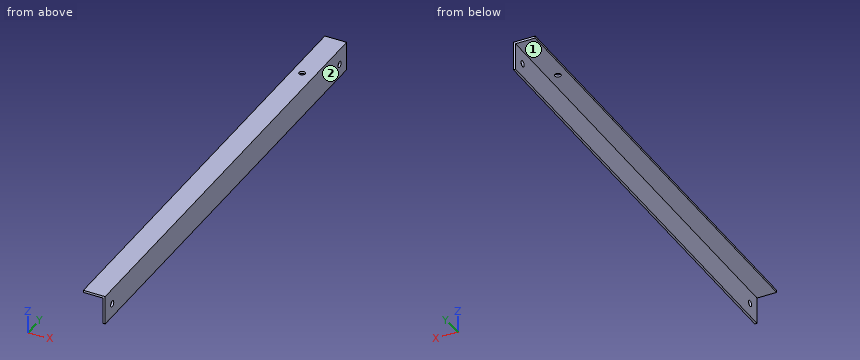
from build123d import *

# Parameters (mm, degrees)
BOX007_W      = 15
BOX007_H      = 317
BOX007_DEPTH  = 20
BOX006_W      = 15
BOX006_H      = 317
BOX006_DEPTH  = 20
SKETCH010_R   = 2.05
HOLE005_DEPTH = 637.469553
SKETCH019_R   = 2.05
HOLE012_DEPTH = 20.001


with BuildPart() as cut017:
    # Box007 → Box007 (new body)
    with BuildSketch(Plane(origin=(1.5, 0, -1.5), x_dir=(1, 0, 0), z_dir=(0, 0, 1))):
        with Locations((7.5, 158.5)):
            Rectangle(BOX007_W, BOX007_H)
    extrude(amount=BOX007_DEPTH)


with BuildPart() as side_middle_body:
    # Box006 → Box006 (new body)
    with BuildSketch(Plane.XY):
        with Locations((7.5, 158.5)):
            Rectangle(BOX006_W, BOX006_H)
    extrude(amount=BOX006_DEPTH)

    # Cut013: cut Cut017
    add(cut017.part, mode=Mode.SUBTRACT)


with BuildPart() as side_middle_body_1:
    # Cut013 placement: moved
    add(side_middle_body.part.moved(Location((1.5, 1.5, 158))))


with BuildPart() as side_middle_body_2:
    # BaseFeature004 placement: moved
    add(side_middle_body_1.part.moved(Location((-1.5, -1.5, -158))))

    # Sketch010 → Hole005 (cut, through all)
    with BuildSketch(Plane.YZ.offset(1.5)):
        with Locations((9.25, 9.25)):
            Circle(SKETCH010_R)
    hole005 = extrude(amount=-HOLE005_DEPTH, mode=Mode.SUBTRACT)

    # Mirrored003: Hole005 across Sketch010 Axis0
    add(hole005.mirror(Plane(origin=(1.5, 158.5, 18.5), x_dir=(1, 0, 0), z_dir=(0, 1, 0))), mode=Mode.SUBTRACT)

    # Sketch019 → Hole012 (cut, through all)
    with BuildSketch(Plane.XY.offset(20)):
        with Locations((8.25, 274.25)):
            Circle(SKETCH019_R)
    extrude(amount=-HOLE012_DEPTH, mode=Mode.SUBTRACT)


with BuildPart() as side_middle_body_3:
    # Body004 placement: moved
    add(side_middle_body_2.part.moved(Location((1.5, 1.5, 169.5))))


with BuildPart() as left_middle_mirror:
    # Part__Mirroring003: instance of side_middle_body
    add(side_middle_body_3.part.mirror(Plane(origin=(1.5e-05, 160, 169.5), x_dir=(0, -1, 0), z_dir=(1, 0, 0))))


with BuildPart() as left_middle_mirror_1:
    # Part__Mirroring003 placement: moved
    add(left_middle_mirror.part.moved(Location((640, 0, 0))))


solid = left_middle_mirror_1.part
Design review of the part built by this model. Coordinates are the model's own, in mm. Face numbers are marked on the shaded views. A direction names the side the tool comes from. Coordinates: 2 decimals unless noted, no trailing zeros. Order: outer loops, then holes, each group sorted by start corner. A loop starts at its lowest first (then second) coordinate and runs counter-clockwise, first axis right, second up. Notation, with made-up numbers: M 32,21.5 L 89,21.5 A30 cw 89,45.5 Z; hole C 9,6 d7. An arc over 180 degrees is marked long. Use a Markdown table: item, result.
(1) For P1, Ø1.5, axis at x = 632.5, y = 66.5, coming from the -Z side; P2, Ø4.5, axis at y = 309.25, z = 178.75, coming from the +X side; P3, Ø4, axis at y = 136.5, z = 179, coming from the -X side, all flat-tipped, find the tip position at first contact; note any pin that passes through.
Worked answers:
| item | result |
|---|---|
| P1 | stops at z = 188 |
| P2 | stops at x = 638.5 |
| P3 | stops at x = 637 |
(2) Wall thickness on probe 1 along Y at (x, z) = (637.85, 178.75); probe 2 along X at (y, z) = (275.75, 188.6); probe 3 along Z at (x, y) = (637.4, 309.25): over which ranges is each line inside the solid? List them lowest first.
Worked answers:
| item | result |
|---|---|
| probe 1 | y = 1.5 to 8.7, 12.8 to 307.2, 311.3 to 318.5 |
| probe 2 | x = 623.5 to 628.2, 632.3 to 638.5 |
| probe 3 | z = 169.5 to 176.7, 180.8 to 189.5 |
(3) Add section A-A (y = 82). Give the boundary of the cut face in (x, z).
Worked answers:
| item | result |
|---|---|
| outline | M 623.5,188 L 637,188 L 637,169.5 L 638.5,169.5 L 638.5,189.5 L 623.5,189.5 Z |
(4) For the marked faces 1 and 2, list the 3-axis set-ups (+Z, -Z, +X, -X, +Y, -Y) from which the entire face can be reached by the end or side of a thin tool; tool diameter is ignored.
Worked answers:
| item | result |
|---|---|
| face 1 | -Z, -X, +Y, -Y |
| face 2 | +Z, -Z, +X, +Y, -Y |
(5) Add section B-B (z = 174). Give the boundary of the cut face in (x, y).
Worked answers:
| item | result |
|---|---|
| outline | M 637,1.5 L 638.5,1.5 L 638.5,318.5 L 637,318.5 Z |
